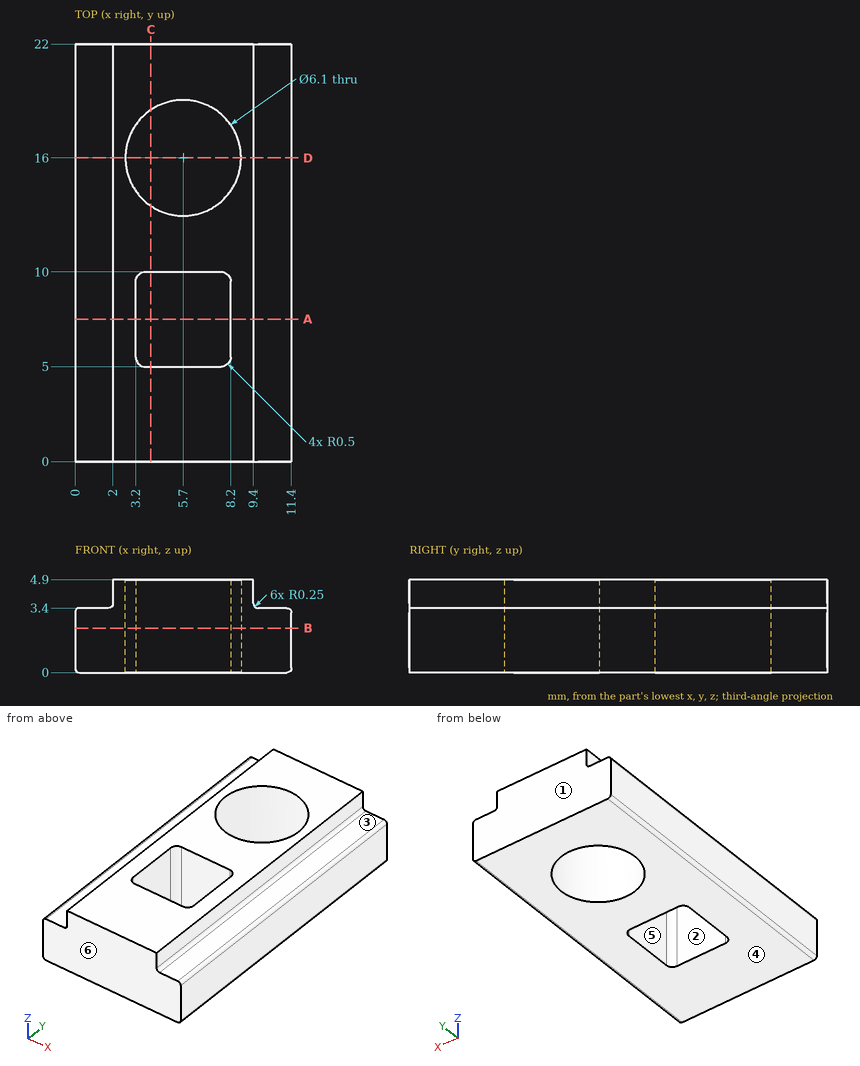
Can you work these out from the drawing? Everything is in mm from the part's minimum corner. A direction names the side the tool comes from. Round coordinates to 2 decimals unless told otherwise and drop trailing zeros. Write each loop counter-clockwise with the first axis right and the second up, starting at its lowest first coordinate (ties: lowest second). Pieces come first, ordered by that corner, then holes.
1. Suppose I cut it at D-D (y = 16). List the corners of the cut face in (x, z) for me.
2. I need wall thicknesses on L1, parallel to Y at x = 5.7, z = 2.15; L2, parallel to Y at x = 4.75, z = 2.65; L3, parallel to X at y = 7, z = 3.1. Which ranges of each line are inside material? Lowest first, please.
3. Suppose I cut it at B-B (z = 2.35). List the corners of the cut face in (x, y) for me.
4. Suppose I cut it at A-A (y = 7.5). List the corners of the cut face in (x, z) for me, and give its area (3 significant figures).
5. Suppose I cut it at C-C (x = 4). List the corners of the cut face in (y, z) for me, and give its area (3 significant figures).
6. Will these pins go through, and if not, where does the flat tip stop? pin 1 Ø1.2 at (x, y) = (10.5, 10) entering from +Z; pin 2 Ø2 at (y, z) = (7, 1.5) entering from -X; pin 3 Ø1 at (y, z) = (7.5, 4.5) entering from -X.
7. For the marked faces 1, 2 and 3, which set-ups out of +Z, -Z, +X, -X, +Y, -Y let a thin tool reach every point of the face, with its end or its side?
8. If we mould it in two halves opening along Y, with no side actions, what happens to the marked faces 4, 5 and 6? For each: released by +Y, released by -Y, zero draft, split by the parting line, or undercut.
Answer sheet:
1. outline: (0, 0.25) arc R0.25 ccw to (0.25, 0) - (2.65, 0) - (2.65, 4.9) - (2, 4.9) - (2, 3.65) arc R0.25 cw to (1.75, 3.4) - (0.25, 3.4) arc R0.25 ccw to (0, 3.15) - close; (8.75, 0) - (11.15, 0) arc R0.25 ccw to (11.4, 0.25) - (11.4, 3.15) arc R0.25 ccw to (11.15, 3.4) - (9.65, 3.4) arc R0.25 cw to (9.4, 3.65) - (9.4, 4.9) - (8.75, 4.9) - close
2. L1: y = 0 to 5, 10 to 12.95, 19.05 to 22
2. L2: y = 0 to 5, 10 to 13.1, 18.9 to 22
2. L3: x = 0 to 3.2, 8.2 to 11.4
3. outline: (0, 0) - (11.4, 0) - (11.4, 22) - (0, 22) - close; hole circle Ø6.1 at (5.7, 16); hole (3.2, 5.5) arc R0.5 ccw to (3.7, 5) - (7.7, 5) arc R0.5 ccw to (8.2, 5.5) - (8.2, 9.5) arc R0.5 ccw to (7.7, 10) - (3.7, 10) arc R0.5 ccw to (3.2, 9.5) - close
4. outline: (0, 0.25) arc R0.25 ccw to (0.25, 0) - (3.2, 0) - (3.2, 4.9) - (2, 4.9) - (2, 3.65) arc R0.25 cw to (1.75, 3.4) - (0.25, 3.4) arc R0.25 ccw to (0, 3.15) - close; (8.2, 0) - (11.15, 0) arc R0.25 ccw to (11.4, 0.25) - (11.4, 3.15) arc R0.25 ccw to (11.15, 3.4) - (9.65, 3.4) arc R0.25 cw to (9.4, 3.65) - (9.4, 4.9) - (8.2, 4.9) - close
4. area: 25.3 mm2
5. outline: (0, 0) - (5, 0) - (5, 4.9) - (0, 4.9) - close; (10, 0) - (13.47, 0) - (13.47, 4.9) - (10, 4.9) - close; (18.53, 0) - (22, 0) - (22, 4.9) - (18.53, 4.9) - close
5. area: 58.5 mm2
6. pin 1: stops at z = 3.4
6. pin 2: stops at x = 0
6. pin 3: stops at x = 2
7. face 1: +Z, -Z, +X, -X, +Y
7. face 2: +Z, -Z
7. face 3: +Z, +X, +Y, -Y
8. face 4: zero draft
8. face 5: undercut
8. face 6: released by -Y
